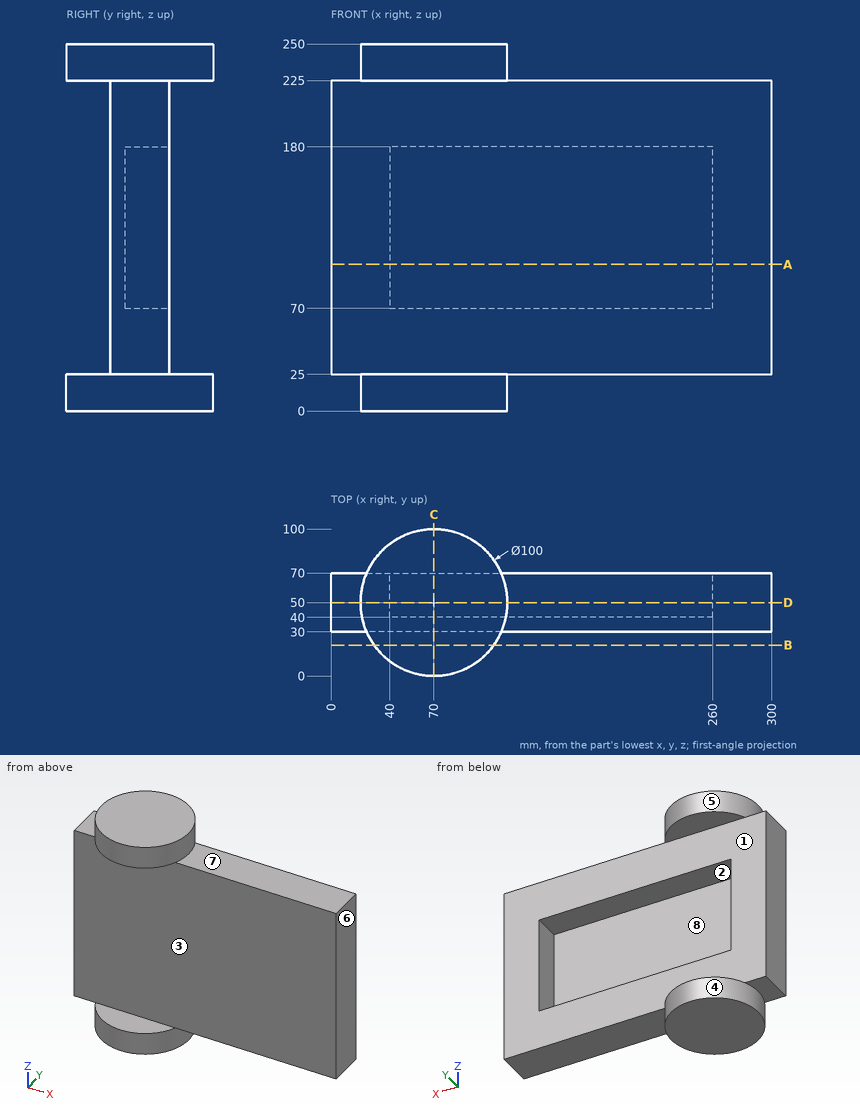
Source: three-view drawing plus pictorial views. Frame: mm from the lowest corner of the part. A direction names the side the tool comes from. Give positions to 0.01 mm unless a question says otherwise; leave off trailing zeros. Loops run counter-clockwise (first coordinate to the right, second up) from the corner with the lowest first, then second, coordinate; pieces in that order, holes last.
1) Section query A-A on z = 100. Return the cut outline in (x, y), and give its area (3 significant figures).
A:
outline: (0, 30) - (300, 30) - (300, 70) - (260, 70) - (260, 40) - (40, 40) - (40, 70) - (0, 70) - close
area: 5,400 mm2
2) Section query B-B on y = 21. Return the cut outline in (x, z).
A:
outline: (29.27, 0) - (110.73, 0) - (110.73, 25) - (29.27, 25) - close; (29.27, 225) - (110.73, 225) - (110.73, 250) - (29.27, 250) - close
3) Reachability of the marked faces 1, 2, 3, 4 and 5 from +Z, -Z, +X, -X, +Y, -Y: full face, straight path, thin tool, end or side. Return the list, or none.
A:
face 1: +X, -X, +Y
face 2: +Y
face 3: +X, -X, -Y
face 4: -Z
face 5: +Z
4) Mould query, pull axis X, two halves, no side actions, for the marked faces 6, 7 and 8. Classes: released by +X, released by -X, zero draft, split by the parting line, or undercut.
A:
face 6: released by +X
face 7: zero draft
face 8: undercut
5) Line query: L1, parallel to X at y = 56, z = 91; L2, parallel to Z at x = 186, y = 51.5; L3, parallel to Z at x = 59, y = 7. Output: solid intervals per line, ascending.
A:
L1: x = 0 to 40, 260 to 300
L2: z = 25 to 70, 180 to 225
L3: z = 0 to 25, 225 to 250
6) Section query C-C on x = 70. Return the cut outline in (y, z).
A:
outline: (0, 0) - (100, 0) - (100, 25) - (70, 25) - (70, 70) - (40, 70) - (40, 180) - (70, 180) - (70, 225) - (100, 225) - (100, 250) - (0, 250) - (0, 225) - (30, 225) - (30, 25) - (0, 25) - close
7) Contact query for flat-ended pins moving along their axis: pin 1 (7.5 mm diameter, centred on x = 18, y = 41, fed in from -Z); pin 2 (20 mm diameter, centred on x = 171.5, y = 54, fed in from +Z); pin 3 (1.5 mm diameter, centred on x = 72, z = 99, fed in from -Y); pin 4 (6 mm diameter, centred on x = 151, z = 104, fed in from +Y). Output: stop coordinate, or through.
A:
pin 1: stops at z = 0
pin 2: stops at z = 225
pin 3: stops at y = 30
pin 4: stops at y = 40
8) Section query D-D on y = 50. Return the cut outline in (x, z).
A:
outline: (0, 25) - (20, 25) - (20, 0) - (120, 0) - (120, 25) - (300, 25) - (300, 225) - (120, 225) - (120, 250) - (20, 250) - (20, 225) - (0, 225) - close; hole (40, 70) - (260, 70) - (260, 180) - (40, 180) - close
